```python
from build123d import *

# Parameters (mm, degrees)
SKETCH1_R           = 1.5
BOSS_EXTRUDE1_DEPTH = 2
SKETCH2_R           = 18.25
BOSS_EXTRUDE2_DEPTH = 17.5
SKETCH3_R           = 8
BOSS_EXTRUDE3_DEPTH = 2
SKETCH4_R           = 2.5
BOSS_EXTRUDE4_DEPTH = 13
CUT_EXTRUDE1_START  = -10
CUT_EXTRUDE1_DEPTH  = 10


with BuildPart() as part:
    # Sketch1 → Boss-Extrude1 (new body)
    with BuildSketch(Plane.XY):
        with BuildLine():
            Line((-23.244095226, 4.829629131), (-17.058114991, 6.48715754))
            ThreePointArc((-17.058114991, 6.48715754), (0, 18.25), (17.058114991, 6.48715754))
            Line((17.058114991, 6.48715754), (23.244095226, 4.829629131))
            ThreePointArc((23.244095226, 4.829629131), (26.95, 0), (23.244095226, -4.829629131))
            Line((23.244095226, -4.829629131), (17.058114991, -6.48715754))
            ThreePointArc((17.058114991, -6.48715754), (0, -18.25), (-17.058114991, -6.48715754))
            Line((-17.058114991, -6.48715754), (-23.244095226, -4.829629131))
            ThreePointArc((-23.244095226, -4.829629131), (-26.95, 0), (-23.244095226, 4.829629131))
        make_face()
        with Locations((-21.95, 0)):
            Circle(SKETCH1_R, mode=Mode.SUBTRACT)
        with Locations((21.95, 0)):
            Circle(SKETCH1_R, mode=Mode.SUBTRACT)
    extrude(amount=-BOSS_EXTRUDE1_DEPTH)

    # Sketch2 → Boss-Extrude2 (add)
    with BuildSketch(Plane(origin=(0, 0, -2), x_dir=(-1, 0, 0), z_dir=(0, 0, -1))):
        with Locations(Location((0, 0, 0), (0, 0, 200.821681464))):
            Circle(SKETCH2_R)
    extrude(amount=BOSS_EXTRUDE2_DEPTH)

    # Sketch3 → Boss-Extrude3 (add)
    with BuildSketch(Plane.XY):
        Circle(SKETCH3_R)
    extrude(amount=BOSS_EXTRUDE3_DEPTH)

    # Sketch4 → Boss-Extrude4 (add)
    with BuildSketch(Plane.XY.offset(2)):
        with Locations(Location((0, 0, 0), (0, 0, 180))):
            Circle(SKETCH4_R)
    extrude(amount=BOSS_EXTRUDE4_DEPTH)

    # Sketch5 → Cut-Extrude1 (cut)
    with BuildSketch(Plane.XY.offset(15).offset(CUT_EXTRUDE1_START)):
        with BuildLine():
            Line((1.5, 2), (-1.5, 2))
            ThreePointArc((-1.5, 2), (0, 2.5), (1.5, 2))
        make_face()
    extrude(amount=CUT_EXTRUDE1_DEPTH, mode=Mode.SUBTRACT)


solid = part.part
```
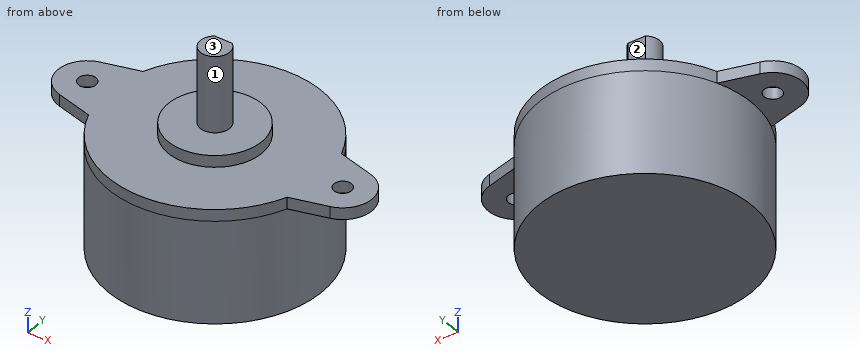
Input: part model. Units: mm. Frame: model coordinates. Face numbers are marked on the shaded views. A direction names the side the tool comes from. Round coordinates to 2 decimals unless told otherwise and drop trailing zeros. Write each loop counter-clockwise with the first axis right and the second up, starting at its lowest first coordinate (ties: lowest second). Pieces come first, ordered by that corner, then holes. Notation, with made-up numbers: (-12.75, 25.25) - (31.25, 25.25) arc R21 ccw to (31.25, 30.25) - close; hole circle Ø9 at (-2, 68). An arc over 180 degrees is marked (long way). Write item = value, one per line.
(1) Contact query for flat-ended pins moving along their axis: pin 1 Ø3 at (x, y) = (7.5, 12.5) entering from +Z; pin 2 Ø6 at (x, y) = (-4.5, -5.5) entering from +Z; pin 3 Ø6 at (y, z) = (10, -0.5) entering from +X. Output: stop coordinate, or through.
Geometry check:
pin_1 = 0
pin_2 = 2
pin_3 = 16.85
(2) Section query C-C on x = 0. Output: boundary loops of the cut face in (y, z).
Geometry check:
outline = (-18.25, -19.5) - (18.25, -19.5) - (18.25, 0) - (8, 0) - (8, 2) - (2.5, 2) - (2.5, 5) - (2, 5) - (2, 15) - (-2.5, 15) - (-2.5, 2) - (-8, 2) - (-8, 0) - (-18.25, 0) - close
(3) Section query B-B on x = 21.95. Output: boundary loops of the cut face in (y, z).
Geometry check:
outline = (-5.18, -2) - (-1.5, -2) - (-1.5, 0) - (-5.18, 0) - close; (1.5, -2) - (5.18, -2) - (5.18, 0) - (1.5, 0) - close
(4) Material intervals for probe 1 along Z at (x, y) = (1, -11); probe 2 along Z at (x, y) = (0, 5.5); probe 3 along Y at (x, z) = (21.95, -1.2), sorted ascending.
Geometry check:
probe_1 = -19.5 to 0
probe_2 = -19.5 to 2
probe_3 = -5.18 to -1.5, 1.5 to 5.18
(5) Section query A-A on y = 0. Output: boundary loops of the cut face in (x, z).
Geometry check:
outline = (-26.95, -2) - (-23.45, -2) - (-23.45, 0) - (-26.95, 0) - close; (-20.45, -2) - (-18.25, -2) - (-18.25, -19.5) - (18.25, -19.5) - (18.25, -2) - (20.45, -2) - (20.45, 0) - (8, 0) - (8, 2) - (2.5, 2) - (2.5, 15) - (-2.5, 15) - (-2.5, 2) - (-8, 2) - (-8, 0) - (-20.45, 0) - close; (23.45, -2) - (26.95, -2) - (26.95, 0) - (23.45, 0) - close
(6) Section query D-D on y = -5.5. Output: boundary loops of the cut face in (x, z).
Geometry check:
outline = (-20.74, -2) - (-17.4, -2) - (-17.4, -19.5) - (17.4, -19.5) - (17.4, -2) - (20.74, -2) - (20.74, 0) - (5.81, 0) - (5.81, 2) - (-5.81, 2) - (-5.81, 0) - (-20.74, 0) - close
(7) Access query for the marked faces 1, 2 and 3. Directions: +Z, -Z, +X, -X, +Y, -Y. A direction counts if a zero-diameter tool reaches every point of the face in a straight line with its end or side. Return the directions, or none.
Geometry check:
face_1 = +Z
face_2 = +Z, +X, -X, +Y
face_3 = +Z, +X, -X, +Y, -Y
